For this review, take the finished solid that the model builds, in its own axes (mm). Face numbers are marked on the shaded views. A direction names the side the tool comes from. Round coordinates to 2 decimals unless told otherwise and drop trailing zeros. Order: outer loops, then holes, each group sorted by start corner. A loop starts at its lowest first (then second) coordinate and runs counter-clockwise, first axis right, second up. Notation, with made-up numbers: (-27, -11.75) - (-18, -11.75) arc R19 ccw to (-18, -2.75) - close; hole circle Ø10 at (0, 8.5). An arc over 180 degrees is marked (long way). One line per question, with ' | ' between items.
```python
from build123d import *

# Parameters (mm, degrees)
F0_R     = 10
F1_DEPTH = 4.55
F2_R     = 2.4
F3_DEPTH = 2.5
F4_DEPTH = 25
F5_DEPTH = 0.6
F6_R     = 3.825
F6_R_2   = 3.125
F7_DEPTH = 0.65


with BuildPart() as f1:
    # F0 (on Top) → F1 (new body)
    with BuildSketch(Plane.XY):
        Circle(F0_R)
    extrude(amount=F1_DEPTH)

    # F2 (on face) → F3 (cut)
    with BuildSketch(Plane(origin=(0, 0, 0), x_dir=(1, 0, 0), z_dir=(0, 0, -1))):
        with BuildLine():
            ThreePointArc((5.1166810842, 0.45), (6.1969215277, 2.0588121749), (8.1080149502, 2.3796204672))
            ThreePointArc((8.1080149502, 2.3796204672), (5.975052301, 5.975052301), (2.3796204672, 8.1080149502))
            ThreePointArc((2.3796204672, 8.1080149502), (2.4323414794, 7.818623786), (2.45, 7.525))
            ThreePointArc((2.45, 7.525), (1.8848076825, 5.9597524158), (0.45, 5.1166810842))
            Line((0.45, 5.1166810842), (0.45, 3.9242833741))
            ThreePointArc((0.45, 3.9242833741), (2.7930717857, 2.7930717857), (3.9242833741, 0.45))
            Line((3.9242833741, 0.45), (5.1166810842, 0.45))
        make_face()
        with BuildLine():
            ThreePointArc((-0.45, 5.1166810842), (-2.0588121749, 6.1969215277), (-2.3796204672, 8.1080149502))
            ThreePointArc((-2.3796204672, 8.1080149502), (-5.975052301, 5.975052301), (-8.1080149502, 2.3796204672))
            ThreePointArc((-8.1080149502, 2.3796204672), (-6.1969215277, 2.0588121749), (-5.1166810842, 0.45))
            Line((-5.1166810842, 0.45), (-3.9242833741, 0.45))
            ThreePointArc((-3.9242833741, 0.45), (-2.7930717857, 2.7930717857), (-0.45, 3.9242833741))
            Line((-0.45, 3.9242833741), (-0.45, 5.1166810842))
        make_face()
        with BuildLine():
            ThreePointArc((-8.1080149502, -2.3796204672), (-5.975052301, -5.975052301), (-2.3796204672, -8.1080149502))
            ThreePointArc((-2.3796204672, -8.1080149502), (-2.0588121749, -6.1969215277), (-0.45, -5.1166810842))
            Line((-0.45, -5.1166810842), (-0.45, -3.9242833741))
            ThreePointArc((-0.45, -3.9242833741), (-2.7930717857, -2.7930717857), (-3.9242833741, -0.45))
            Line((-3.9242833741, -0.45), (-5.1166810842, -0.45))
            ThreePointArc((-5.1166810842, -0.45), (-6.1969215277, -2.0588121749), (-8.1080149502, -2.3796204672))
        make_face()
        with BuildLine():
            ThreePointArc((2.3796204672, -8.1080149502), (5.975052301, -5.975052301), (8.1080149502, -2.3796204672))
            ThreePointArc((8.1080149502, -2.3796204672), (6.1969215277, -2.0588121749), (5.1166810842, -0.45))
            Line((5.1166810842, -0.45), (3.9242833741, -0.45))
            ThreePointArc((3.9242833741, -0.45), (2.7930717857, -2.7930717857), (0.45, -3.9242833741))
            Line((0.45, -3.9242833741), (0.45, -5.1166810842))
            ThreePointArc((0.45, -5.1166810842), (1.8848076825, -5.9597524158), (2.45, -7.525))
            ThreePointArc((2.45, -7.525), (2.4323414794, -7.818623786), (2.3796204672, -8.1080149502))
        make_face()
        with BuildLine():
            ThreePointArc((8.3331614938, -0.45), (8.420314018, -0.2324603388), (8.45, 0))
            ThreePointArc((8.45, 0), (8.420314018, 0.2324603388), (8.3331614938, 0.45))
            ThreePointArc((8.3331614938, 0.45), (6.6, 0), (8.3331614938, -0.45))
        make_face()
        with BuildLine():
            ThreePointArc((-8.3331614938, 0.45), (-8.4203140187, 0.2324603363), (-8.45, -5.3e-09))
            ThreePointArc((-8.45, -5.3e-09), (-8.4203140174, -0.2324603414), (-8.3331614938, -0.45))
            ThreePointArc((-8.3331614938, -0.45), (-7.2925396612, -0.895314018), (-6.6, 0))
            ThreePointArc((-6.6, 0), (-7.2925396612, 0.895314018), (-8.3331614938, 0.45))
        make_face()
        with BuildLine():
            ThreePointArc((0.45, 8.3331614938), (0.2324603388, 8.420314018), (0, 8.45))
            ThreePointArc((0, 8.45), (-0.2324603388, 8.420314018), (-0.45, 8.3331614938))
            ThreePointArc((-0.45, 8.3331614938), (-0.4687083315, 6.7275431046), (0.925, 7.525))
            ThreePointArc((0.925, 7.525), (0.7974568954, 7.9937083315), (0.45, 8.3331614938))
        make_face()
        with BuildLine():
            ThreePointArc((-0.45, -8.3331614938), (-0.2324603347, -8.4203140191), (8.6e-09, -8.45))
            ThreePointArc((8.6e-09, -8.45), (0.232460343, -8.4203140169), (0.45, -8.3331614938))
            ThreePointArc((0.45, -8.3331614938), (0.7974568954, -7.9937083315), (0.925, -7.525))
            ThreePointArc((0.925, -7.525), (-0.4687083315, -6.7275431046), (-0.45, -8.3331614938))
        make_face()
        Circle(F2_R)
    extrude(amount=-F3_DEPTH, mode=Mode.SUBTRACT)

    # F4 (cut): faces of the model
    f4_faces = [f1.faces().sort_by_distance(p)[0] for p in [
        (7.525, 0, 2.5),
        (-7.525, 0, 2.5),
        (0, -7.525, 2.5),
        (0, 0, 2.5),
        (0, 7.525, 2.5),
    ]]
    extrude(f4_faces, amount=-F4_DEPTH, mode=Mode.SUBTRACT)

    # F2 (on face) → F5 (cut)
    with BuildSketch(Plane(origin=(0, 0, 0), x_dir=(1, 0, 0), z_dir=(0, 0, -1))):
        with BuildLine():
            ThreePointArc((3.95, 0), (3.9435656028, 0.2253671143), (3.9242833741, 0.45))
            ThreePointArc((3.9242833741, 0.45), (2.7930717857, 2.7930717857), (0.45, 3.9242833741))
            ThreePointArc((0.45, 3.9242833741), (0, 3.95), (-0.45, 3.9242833741))
            ThreePointArc((-0.45, 3.9242833741), (-2.7930717857, 2.7930717857), (-3.9242833741, 0.45))
            ThreePointArc((-3.9242833741, 0.45), (-3.95, 0), (-3.9242833741, -0.45))
            ThreePointArc((-3.9242833741, -0.45), (-2.7930717857, -2.7930717857), (-0.45, -3.9242833741))
            ThreePointArc((-0.45, -3.9242833741), (0, -3.95), (0.45, -3.9242833741))
            ThreePointArc((0.45, -3.9242833741), (2.7930717857, -2.7930717857), (3.9242833741, -0.45))
            ThreePointArc((3.9242833741, -0.45), (3.9435656028, -0.2253671143), (3.95, 0))
        make_face()
        Circle(F2_R, mode=Mode.SUBTRACT)
        with BuildLine():
            Line((0.45, 3.9242833741), (0.45, 5.1166810842))
            ThreePointArc((0.45, 5.1166810842), (0, 5.075), (-0.45, 5.1166810842))
            Line((-0.45, 5.1166810842), (-0.45, 3.9242833741))
            ThreePointArc((-0.45, 3.9242833741), (0, 3.95), (0.45, 3.9242833741))
        make_face()
        with BuildLine():
            ThreePointArc((5.1166810842, -0.45), (5.075, 0), (5.1166810842, 0.45))
            Line((5.1166810842, 0.45), (3.9242833741, 0.45))
            ThreePointArc((3.9242833741, 0.45), (3.9435656028, 0.2253671143), (3.95, 0))
            ThreePointArc((3.95, 0), (3.9435656028, -0.2253671143), (3.9242833741, -0.45))
            Line((3.9242833741, -0.45), (5.1166810842, -0.45))
        make_face()
        with BuildLine():
            Line((-0.45, -3.9242833741), (-0.45, -5.1166810842))
            ThreePointArc((-0.45, -5.1166810842), (0, -5.075), (0.45, -5.1166810842))
            Line((0.45, -5.1166810842), (0.45, -3.9242833741))
            ThreePointArc((0.45, -3.9242833741), (0, -3.95), (-0.45, -3.9242833741))
        make_face()
        with BuildLine():
            Line((-3.9242833741, 0.45), (-5.1166810842, 0.45))
            ThreePointArc((-5.1166810842, 0.45), (-5.0854425254, 0.2259631125), (-5.075, 0))
            ThreePointArc((-5.075, 0), (-5.0854425254, -0.2259631125), (-5.1166810842, -0.45))
            Line((-5.1166810842, -0.45), (-3.9242833741, -0.45))
            ThreePointArc((-3.9242833741, -0.45), (-3.95, 0), (-3.9242833741, 0.45))
        make_face()
    extrude(amount=-F5_DEPTH, mode=Mode.SUBTRACT)

    # F6 (on face) → F7 (join)
    with BuildSketch(Plane.XY.offset(4.55)):
        Circle(F6_R)
        Circle(F6_R_2, mode=Mode.SUBTRACT)
    extrude(amount=F7_DEPTH)


solid = f1.part
```
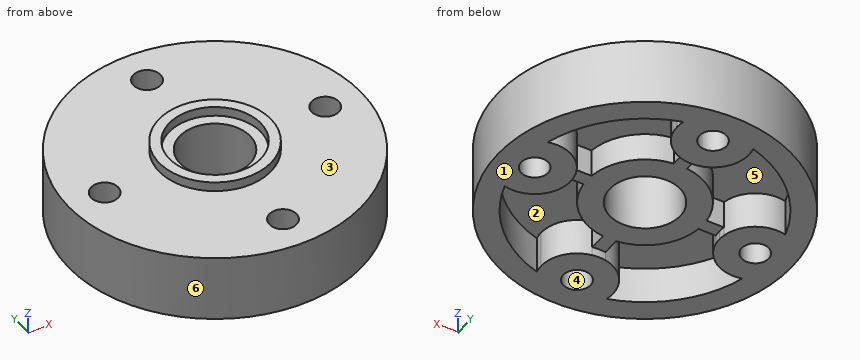
(1) For probe 1 along X at (y, z) = (6, 0.85); probe 2 along X at (y, z) = (-6.5, 0.45); probe 3 along X at (y, z) = (2, 0.8), list the stretches that pass through material, from the lowest coordinate up. Write a range as [from, to].
Output values:
probe 1: [-8, -5.95], [-1.92, 1.92], [5.95, 8] | probe 2: [-7.6, -5.4], [-2.23, 2.23], [5.4, 7.6] | probe 3: [-9.8, -6.11], [-3.41, -1.33], [1.33, 3.41], [6.11, 9.8]
(2) We need section C-C on z = 2.2. Give the number of separate pieces and of enclosed holes in the cut face, plus the area to 3 significant figures.
Output values:
separate pieces: 1 | enclosed holes: 9 | area: 168 mm^2
(3) We need section B-B on y = 7. State the section outline as (x, z) points.
Output values:
outline: (-7.14, 0) - (-4.73, 0) - (-4.73, 2.5) - (-2.39, 2.5) - (-2.39, 0) - (-0.76, 0) - (-0.76, 4.55) - (-7.14, 4.55) - close; (0.76, 0) - (2.39, 0) - (2.39, 2.5) - (4.73, 2.5) - (4.73, 0) - (7.14, 0) - (7.14, 4.55) - (0.76, 4.55) - close
(4) For the marked faces 1 and 2, list the 3-axis set-ups (+Z, -Z, +X, -X, +Y, -Y) from which the entire face can be reached by the end or side of a thin tool; tool diameter is ignored.
Output values:
face 1: -Z, +X, -X, +Y, -Y | face 2: -Z
(5) We need section D-D on x = -7.5. State the section outline as (y, z) points.
Output values:
outline: (-6.61, 0) - (-3.89, 0) - (-3.89, 2.5) - (-2.45, 2.5) - (-2.45, 0) - (-0.92, 0) - (-0.92, 4.55) - (-6.61, 4.55) - close; (0.92, 0) - (2.45, 0) - (2.45, 2.5) - (3.89, 2.5) - (3.89, 0) - (6.61, 0) - (6.61, 4.55) - (0.92, 4.55) - close
(6) We need section A-A on x = 0. State the section outline as (y, z) points (3 decimals), plus the area to 3 significant figures.
Output values:
outline: (-10, 0) - (-8.45, 0) - (-8.45, 4.55) - (-10, 4.55) - close; (-6.6, 0) - (-5.075, 0) - (-5.075, 0.6) - (-2.4, 0.6) - (-2.4, 4.55) - (-3.125, 4.55) - (-3.125, 5.2) - (-3.825, 5.2) - (-3.825, 4.55) - (-6.6, 4.55) - close; (2.4, 0.6) - (5.075, 0.6) - (5.075, 0) - (6.6, 0) - (6.6, 4.55) - (3.825, 4.55) - (3.825, 5.2) - (3.125, 5.2) - (3.125, 4.55) - (2.4, 4.55) - close; (8.45, 0) - (10, 0) - (10, 4.55) - (8.45, 4.55) - close | area: 50.0 mm^2
(7) Insertion check: pin 1 (7 mm diameter, centred on x = 0, y = 0, fed in from +Z); pin 2 (1.7 mm diameter, centred on x = -7.525, y = 0, fed in from -Z); pin 3 (1 mm diameter, centred on y = 5, z = 1.5, fed in from -X); pin 4 (1 mm diameter, centred on x = -4.5, z = 2, fed in from -Y). Each pin has a flat end and moves straight along its axis. Give the tip position at first contact, or say it passes through.
Output values:
pin 1: z = 5.2 | pin 2: through | pin 3: x = -8.93 | pin 4: y = -9.17
(8) Mouldability with a two-part tool opening along X and no side actions: class the marked faces 3, 4, 5 and 6 as released by +X, released by -X, zero draft, split by the parting line, or undercut.
Output values:
face 3: zero draft | face 4: undercut | face 5: undercut | face 6: split by the parting line
